from build123d import *

# Parameters (mm, degrees)
F0_R        = 3.5
F1_DEPTH    = 80
F2_R        = 6.3298520118
F2_R_2      = 2.5
F3_DEPTH    = 30
F4_S5_R     = 2.5
F4_T6_DEPTH = 7
F5_R        = 3.175
F6_DEPTH    = 17
F7_SIZE     = 1
F8_W        = 9.7203729674
F8_H        = 8.019306697
F8_W_2      = 5.5
F8_H_2      = 5.8197690165
F9_DEPTH    = 5.5


# Not quite as in the source:
# - a fillet or chamfer that OpenCascade refuses, or shapes differently, is made with other operations: its cross-section is extruded or revolved along the edge and cut away or added


with BuildPart() as f1:
    # F0 (on Front) → F1 (new body)
    with BuildSketch(Plane.XZ):
        Circle(F0_R)
    extrude(amount=F1_DEPTH)

    # F2 (on face) → F3 (cut)
    with BuildSketch(Plane.XZ.offset(80)):
        Circle(F2_R)
        Circle(F2_R_2, mode=Mode.SUBTRACT)
    extrude(amount=-F3_DEPTH, mode=Mode.SUBTRACT)

    # F4: chamfer of 2 on 1 edges, made by hand


with BuildPart() as f4_tool2:
    # F4_s3 → F4_t4 (revolve)
    with BuildSketch(Plane.XY):
        Polygon((3.5, -48), (1.5, -50), (3.5, -50), align=None)
    revolve(axis=Axis((0, -50, 0), (0, 1, 0)))

    # F4_s5 → F4_t6 (cut, symmetric)
    with BuildSketch(Plane.XZ.offset(49)):
        Circle(F4_S5_R)
    extrude(amount=F4_T6_DEPTH, both=True, mode=Mode.SUBTRACT)


with BuildPart() as f1_1:
    add(f1.part)

    # F4_t1: cut F4_tool2
    add(f4_tool2.part, mode=Mode.SUBTRACT)

    # F5 (on face) → F6 (join)
    with BuildSketch(Plane.XZ.offset(80)):
        Circle(F5_R)
    extrude(amount=-F6_DEPTH)

    # F7
    f7_edges = [f1_1.edges().sort_by_distance(p)[0] for p in [
        (-3.175, -80, 0),
    ]]
    chamfer(f7_edges, length=F7_SIZE)

    # F8 (on face) → F9 (cut)
    with BuildSketch(Plane(origin=(0, 0, 0), x_dir=(-1, 0, 0), z_dir=(0, 1, 0))):
        Rectangle(F8_W, F8_H)
        Rectangle(F8_W_2, F8_H_2, mode=Mode.SUBTRACT)
    extrude(amount=-F9_DEPTH, mode=Mode.SUBTRACT)


solid = f1_1.part
Model file for the job. Use its own axes, mm. A direction names the side the tool comes from. Give positions to 0.01 mm unless a question says otherwise; leave off trailing zeros. Order: outer loops, then holes, each group sorted by start corner. A loop starts at its lowest first (then second) coordinate and runs counter-clockwise, first axis right, second up. Notation, with made-up numbers: M 29,24.5 L 84,24.5 A23 ccw 84,40.5 Z; hole C 26.5,62 d6. An arc over 180 degrees is marked long. Write item = value, one per line.
Q1. Cut at C-C, the plane y = -34. List the corners of the cut face in (x, z).
Derived:
outline = C 0,0 d7
Q2. Cut at D-D, the plane y = -53. List the corners of the cut face in (x, z), then the cut area to 3 significant figures.
Derived:
outline = C 0,0 d5
area = 19.6 mm2
Q3. Tool access for faces 4 (the flat face through (-2.75, -3, 0)), 5 (the cylindrical face through (-0.69, -71.11, -3.1)), 6 (the flat face through (0, -63, -3)), 7 (the flat face through (0, -3, -2.91)): list every direction of +Z, -Z, +X, -X, +Y, -Y with a clear straight run to the whole face (end or side of a thin tool).
Derived:
face_4 = +Z, -Z, -X, +Y
face_5 = -Y
face_6 = none
face_7 = -Z, +X, -X, +Y
Q4. Drill centre lines: line 1 (Y direction, x = -1.25, z = -2.75); line 2 (X direction, y = -5, z = 2.75); line 3 (Z direction, x = -1.5, y = -41). Where is each one in solid material? Low to high. Write a range as [from, to].
Derived:
line_1 = [-79.15, -63], [-48.48, 0]
line_2 = [-2.17, 2.17]
line_3 = [-3.16, 3.16]
Q5. Flat gauge pins, fed straight in: pin 1 (3 mm diameter, centred on x = -0.5, y = -2.5, fed in from -Z); pin 2 (1 mm diameter, centred on x = -2, y = -35.5, fed in from +Z); pin 3 (1.2 mm diameter, centred on x = -0.5, y = -2, fed in from +Z). Where does each tip first touch, or does it go through?
Derived:
pin_1 = -2.91
pin_2 = 3.16
pin_3 = 2.91
Q6. Cut at B-B, the plane x = 0. List the corners of the cut face in (y, z) (3 decimals), then the cut area to 3 significant figures.
Derived:
outline = M -80,-2.175 L -79,-3.175 L -63,-3.175 L -63,-2.5 L -49,-2.5 L -48,-3.5 L -5.5,-3.5 L -5.5,-2.91 L 0,-2.91 L 0,2.91 L -5.5,2.91 L -5.5,3.5 L -48,3.5 L -49,2.5 L -63,2.5 L -63,3.175 L -79,3.175 L -80,2.175 Z
area = 512 mm2
Q7. Two-plate mould, pull along Y, no slides. Class faces 1 (the flat face through (0, 0, 0)), 2 (the cylindrical face through (-0.54, -56.1, -2.44)), 3 (the cylindrical face through (-2.58, -23.664, 2.365)): pulls with the +Y half, pulls with the -Y half, needs draft (parallel to the pull), parting line crosses it, or undercut.
Derived:
face_1 = pulls with the +Y half
face_2 = undercut
face_3 = needs draft
Q8. Cut at A-A, the plane z = 0. List the corners of the cut face in (x, y) (3 decimals).
Derived:
outline = M -3.5,-48 L -2.5,-49 L -2.5,-63 L -3.175,-63 L -3.175,-79 L -2.175,-80 L 2.175,-80 L 3.175,-79 L 3.175,-63 L 2.5,-63 L 2.5,-49 L 3.5,-48 L 3.5,-5.5 L 2.75,-5.5 L 2.75,0 L -2.75,0 L -2.75,-5.5 L -3.5,-5.5 Z
